```python
from build123d import *

# Parameters (mm, degrees)
F0_R     = 38.1
F2_DEPTH = 123.825
F1_R     = 31.75
F3_DEPTH = 121.92
F4_R     = 5.08
F5_R     = 2.54


with BuildPart() as f2:
    # F0 (on Top) → F2 (new body)
    with BuildSketch(Plane.XY):
        Circle(F0_R)
    extrude(amount=F2_DEPTH)

    # F1 (on Top) → F3 (cut)
    with BuildSketch(Plane.XY):
        Circle(F1_R)
    extrude(amount=F3_DEPTH, mode=Mode.SUBTRACT)

    # F4
    f4_edges = [f2.edges().sort_by_distance(p)[0] for p in [
        (-38.1, 0, 0),
    ]]
    fillet(f4_edges, radius=F4_R)

    # F5
    f5_edges = [f2.edges().sort_by_distance(p)[0] for p in [
        (-38.1, 0, 123.825),
    ]]
    fillet(f5_edges, radius=F5_R)


solid = f2.part
```
The model under review builds one solid part; all positions refer to its coordinate system, in mm. Coordinates: 2 decimals unless noted, no trailing zeros. Write each loop counter-clockwise with the first axis right and the second up, starting at its lowest first coordinate (ties: lowest second). Pieces come first, ordered by that corner, then holes. Notation, with made-up numbers: (52, -39) -> (103, -39) arc R17 ccw to (103, -7) -> close; hole circle Ø1 at (-3.75, 6). An arc over 180 degrees is marked (long way). One line per item, written item: value. Start each with the question number.
Q1. The part is to be moulded in two halves that separate along Y. For faces 1 (the face through (-30.235, -23.183, 62.369)), 2 (the face through (0, 0, 123.825)), 3 (the face through (0, 0, 121.92)), 4 (the face through (-6.883, -30.995, 60.107)), say which applies: +Y half, -Y half, draft (parallel to the pull), parting line (faces both ways), or undercut.
Q2. Add section C-C, the plane z = 64. Give the boundary of the cut face in (x, y).
Q3. Add section A-A, the plane x = 0. Give the boundary of the cut face in (y, z) (3 decimals), then the cut area to 3 significant figures.
Q4. Clearance check with flat-ended pins moving along their axes: P1, Ø10, axis at y = 19, z = 31.5, coming from the +X side; P2, Ø8, axis at y = -14.5, z = 98.5, coming from the -X side; P3, Ø1.5, axis at y = -22, z = 28.5, coming from the +X side. State where each tip first meets the part, or that it passes through.
Q5. To check wall thickness, follow probe 1 along Y at (x, z) = (0, 27); probe 2 along X at (y, z) = (21, 117). State the ranges of each line that lie inside material, in increasing order.
Response:
1. face 1: parting line
1. face 2: draft
1. face 3: undercut
1. face 4: undercut
2. outline: circle Ø76.2 at (0, 0); hole circle Ø63.5 at (0, 0)
3. outline: (-38.1, 5.08) arc R5.08 ccw to (-33.02, 0) -> (-31.75, 0) -> (-31.75, 121.92) -> (31.75, 121.92) -> (31.75, 0) -> (33.02, 0) arc R5.08 ccw to (38.1, 5.08) -> (38.1, 121.285) arc R2.54 ccw to (35.56, 123.825) -> (-35.56, 123.825) arc R2.54 ccw to (-38.1, 121.285) -> close
3. area: 1,680 mm²
4. P1: x = 35.43
4. P2: x = -36.62
4. P3: x = 31.62
5. probe 1: -38.1 to -31.75, 31.75 to 38.1
5. probe 2: -31.79 to -23.81, 23.81 to 31.79
